Input: part model. Units: mm. Frame: model coordinates. A direction names the side the tool comes from. Give positions to 0.01 mm unless a question says otherwise; leave off trailing zeros. Loops run counter-clockwise (first coordinate to the right, second up) from the corner with the lowest first, then second, coordinate; pieces in that order, holes last. Notation, with made-up numbers: (-31, 69) - (16, 69) arc R35 ccw to (16, 102) - close; hole circle Ø6 at (-20, 16). An arc over 180 degrees is marked (long way). Answer as a JSON object with one key per item and string values.
from build123d import *
from build123d.topology import SkipClean

# Parameters (mm, degrees)
SKETCH2_R           = 45.025932087
SKETCH2_R_2         = 1.9685
BOSS_EXTRUDE1_DEPTH = 10.16
SKETCH3_R           = 3.81
CUT_EXTRUDE1_DEPTH  = 3.81
BOSS_EXTRUDE2_START = 10.16
BOSS_EXTRUDE2_DEPTH = 10.16
SKETCH6_R           = 2.032
CUT_EXTRUDE2_DEPTH  = 10.16
CIRPATTERN2_COUNT   = 4


with BuildPart() as part:
    # Sketch2 → Boss-Extrude1 (new body)
    with BuildSketch(Plane.XY):
        Circle(SKETCH2_R)
        with Locations((0, -22.225)):
            Circle(SKETCH2_R_2, mode=Mode.SUBTRACT)
        with Locations((-22.225, 0)):
            Circle(SKETCH2_R_2, mode=Mode.SUBTRACT)
        with Locations((0, 22.225)):
            Circle(SKETCH2_R_2, mode=Mode.SUBTRACT)
        with Locations((22.225, 0)):
            Circle(SKETCH2_R_2, mode=Mode.SUBTRACT)
    extrude(amount=BOSS_EXTRUDE1_DEPTH)

    # Sketch3 → Cut-Extrude1 (cut)
    with BuildSketch(Plane(origin=(0, 0, 0), x_dir=(-1, 0, 0), z_dir=(0, 0, -1))):
        with Locations((0, 22.225)):
            Circle(SKETCH3_R)
        with Locations((22.225, 0)):
            Circle(SKETCH3_R)
        with Locations((0, -22.225)):
            Circle(SKETCH3_R)
        with Locations((-22.225, 0)):
            Circle(SKETCH3_R)
    extrude(amount=-CUT_EXTRUDE1_DEPTH, mode=Mode.SUBTRACT)

    # Sketch5 → Boss-Extrude2 (add)
    with SkipClean():  # the faces are left unmerged after this step: merging them gives an invalid solid
        with BuildSketch(Plane(origin=(0, 0, 0), x_dir=(-1, 0, 0), z_dir=(0, 0, -1)).offset(BOSS_EXTRUDE2_START)):
            with BuildLine():
                Line((41.699931294, 5.08), (41.699931294, -5.08))
                Line((41.699931294, -5.08), (42.560096203, -5.08))
                ThreePointArc((42.560096203, -5.08), (41.806519891, -9.454262714), (40.604604544, -13.727136578))
                Line((40.604604544, -13.727136578), (42.654370672, -14.420097879))
                ThreePointArc((42.654370672, -14.420097879), (45.025932087, 0), (42.654370672, 14.420097879))
                Line((42.654370672, 14.420097879), (40.604604544, 13.727136578))
                ThreePointArc((40.604604544, 13.727136578), (41.806519891, 9.454262714), (42.560096203, 5.08))
                Line((42.560096203, 5.08), (41.699931294, 5.08))
            make_face()
        boss_extrude2 = extrude(amount=-BOSS_EXTRUDE2_DEPTH)

    # Sketch6 → Cut-Extrude2 (cut)
    with SkipClean():  # the faces are left unmerged after this step: merging them gives an invalid solid
        with BuildSketch(Plane(origin=(-41.699931294, 0, 0), x_dir=(0, 0, -1), z_dir=(1, 0, 0))):
            with Locations(Location((5.08, 0, 0), (0, 0, 90))):
                Circle(SKETCH6_R)
        cut_extrude2 = extrude(amount=-CUT_EXTRUDE2_DEPTH, mode=Mode.SUBTRACT)

    # CirPattern2: Boss-Extrude2, Cut-Extrude2 ×4 about axis
    with SkipClean():  # the faces are left unmerged after this step: merging them gives an invalid solid
        cirpattern2_axis = Axis((0, 0, 0), (0, 0, 1))
        add([boss_extrude2.rotate(cirpattern2_axis, i * 360 / CIRPATTERN2_COUNT) for i in range(1, CIRPATTERN2_COUNT)])
        add([cut_extrude2.rotate(cirpattern2_axis, i * 360 / CIRPATTERN2_COUNT) for i in range(1, CIRPATTERN2_COUNT)], mode=Mode.SUBTRACT)


solid = part.part
Item 1: Cut plane A-A (x = 0). Give the number of separate pieces and of enclosed holes in the cut face, then the cut area to 3 significant figures.
Geometry check:
{"separate pieces": "5", "enclosed holes": "0", "area": "847 mm2"}
Item 2: Cut plane D-D (z = 2). Return loops of the section in (x, y) (3 decimals).
Geometry check:
{"outline": "circle Ø90.052 at (0, 0); hole circle Ø7.62 at (-22.225, 0); hole circle Ø7.62 at (0, -22.225); hole circle Ø7.62 at (0, 22.225); hole circle Ø7.62 at (22.225, 0)"}
Item 3: Access query for faces 4 (the face through (-14.078, -41.644, -5.151)), 5 (the face through (-9.39, 41.82, -5.15)), 6 (the face through (-43, 0, -10.16)). Directions: +Z, -Z, +X, -X, +Y, -Y. A direction counts if a zero-diameter tool reaches every point of the face in a straight line with its end or side. Return the directions, or none.
Geometry check:
{"face 4": "-Z, -X", "face 5": "-Z", "face 6": "-Z, +X, -X, +Y, -Y"}
Item 4: Material intervals for line 1 (Y direction, x = 0, z = 7.5); line 2 (Y direction, x = 2, z = 2.5); line 3 (Z direction, x = 44, y = 0), sorted ascending. Write a range as [from, to].
Geometry check:
{"line 1": "y = [-45.03, -24.19], [-20.26, 20.26], [24.19, 45.03]", "line 2": "y = [-44.98, -25.47], [-18.98, 18.98], [25.47, 44.98]", "line 3": "z = [-10.16, -7.11], [-3.05, 10.16]"}
Item 5: Contact query for flat-ended pins moving along their axis: P1, Ø5, axis at x = 22.225, y = 0, coming from the -Z side; P2, Ø5.5, axis at y = 0, z = -5.08, coming from the -X side; P3, Ø1, axis at x = -33, z = 2.5, coming from the -Y side; P4, Ø8, axis at x = 18.5, z = 1, coming from the -Y side. Output: stop coordinate, or through.
Geometry check:
{"P1": "stops at z = 3.81", "P2": "stops at x = -45.03", "P3": "stops at y = -31.16", "P4": "stops at y = -42.63"}
Item 6: Cut plane C-C (y = -11.5). Return loops of the section in (x, z).
Geometry check:
{"outline": "(-43.53, -10.16) - (-41.29, -10.16) - (-41.29, 0) - (41.29, 0) - (41.29, -10.16) - (43.53, -10.16) - (43.53, 10.16) - (-43.53, 10.16) - close"}
Item 7: Mould query, pull axis Y, two halves, no side actions, for faces 1 (the face through (20.26, 0.09, 6.94)), 2 (the face through (-0.265, 43.34, -3.065)), 3 (the face through (-41.62, -14.07, -5.15)). Classes: released by +Y, released by -Y, zero draft, split by the parting line, or undercut.
Geometry check:
{"face 1": "undercut", "face 2": "zero draft", "face 3": "released by -Y"}
